from build123d import *

# Parameters (mm, degrees)
CROQUIS1_W              = 158
CROQUIS1_H              = 158
CROQUIS1_W_2            = 146
CROQUIS1_H_2            = 146
SALIENTE_EXTRUIR1_DEPTH = 1.5
CROQUIS2_W              = 150
CROQUIS2_H              = 150
CROQUIS2_W_2            = 146
CROQUIS2_H_2            = 146
SALIENTE_EXTRUIR2_DEPTH = 2


with BuildPart() as part:
    # Croquis1 → Saliente-Extruir1 (new body)
    with BuildSketch(Plane(origin=(0, 0, 0), x_dir=(1, 0, 0), z_dir=(0, 1, 0))):
        with Locations((73, 73)):
            Rectangle(CROQUIS1_W, CROQUIS1_H)
        with Locations((73, 73)):
            Rectangle(CROQUIS1_W_2, CROQUIS1_H_2, mode=Mode.SUBTRACT)
    extrude(amount=SALIENTE_EXTRUIR1_DEPTH)

    # Croquis2 → Saliente-Extruir2 (add)
    with BuildSketch(Plane(origin=(0, 1.5, 0), x_dir=(1, 0, 0), z_dir=(0, 1, 0))):
        with Locations((73, 73)):
            Rectangle(CROQUIS2_W, CROQUIS2_H)
        with Locations((73, 73)):
            Rectangle(CROQUIS2_W_2, CROQUIS2_H_2, mode=Mode.SUBTRACT)
    extrude(amount=SALIENTE_EXTRUIR2_DEPTH)


solid = part.part
Can you work these out from the model? Positions are in its coordinate system, mm. A direction names the side the tool comes from. Coordinates: 2 decimals unless noted, no trailing zeros. Write each loop counter-clockwise with the first axis right and the second up, starting at its lowest first coordinate (ties: lowest second). Pieces come first, ordered by that corner, then holes. Notation, with made-up numbers: (50.5, 48) - (99.5, 48) arc R17 ccw to (99.5, 74) - close; hole circle Ø4 at (81, 26.5). An arc over 180 degrees is marked (long way). Return JSON: item names as keys, results as strings. Group by question number.
Item 1: If we section it at A-A (z = -19.5): Write out the boundary of the cut face in (x, y).
Item 2: We'd pull the mould along Z, two halves only. Please class faces 3 (the face through (72, 2, 0)), 4 (the face through (67, 1.5, 3)): pulls with the +Z half, pulls with the -Z half, needs draft (parallel to the pull), parting line crosses it, or undercut.
Item 3: Which directions (+Z, -Z, +X, -X, +Y, -Y) give clear straight access to the entire face, cutting with the end or side of a thin tool? Please do faces 1 (the face through (146, 2, -72)), 2 (the face through (67, 0, 3)).
Item 4: If we section it at B-B (x = 58): Write out the boundary of the cut face in (y, z), then the cut area to 3 significant figures.
Item 5: Please list where these lines run through material, in increasing order: probe 1 along Z at (x, y) = (26, 1.6); probe 2 along X at (y, z) = (1.35, -38.5); probe 3 along Z at (x, y) = (102, 0.9).
Item 6: I'm going to push flat-ended pins straight in: pin 1 Ø1.5 at (y, z) = (2.5, -53.5) entering from +X; pin 2 Ø1 at (y, z) = (2.5, -48) entering from -X. Where does each tip first touch, or does it pass through?
Item 7: If we section it at C-C (y = 2.35): Write out the boundary of the cut face in (x, z), then the cut area to 3 significant figures.
Return value:
{
 "1": {"outline": "(-6, 0) - (0, 0) - (0, 3.5) - (-2, 3.5) - (-2, 1.5) - (-6, 1.5) - close; (146, 0) - (152, 0) - (152, 1.5) - (148, 1.5) - (148, 3.5) - (146, 3.5) - close"},
 "2": {"face 3": "undercut", "face 4": "needs draft"},
 "3": {"face 1": "+Y, -Y", "face 2": "+Z, -Z, +X, -X, -Y"},
 "4": {"outline": "(0, -152) - (1.5, -152) - (1.5, -148) - (3.5, -148) - (3.5, -146) - (0, -146) - close; (0, 0) - (3.5, 0) - (3.5, 2) - (1.5, 2) - (1.5, 6) - (0, 6) - close", "area": "26.0 mm^2"},
 "5": {"probe 1": "z = -148 to -146, 0 to 2", "probe 2": "x = -6 to 0, 146 to 152", "probe 3": "z = -152 to -146, 0 to 6"},
 "6": {"pin 1": "stops at x = 148", "pin 2": "stops at x = -2"},
 "7": {"outline": "(-2, -148) - (148, -148) - (148, 2) - (-2, 2) - close; hole (0, -146) - (146, -146) - (146, 0) - (0, 0) - close", "area": "1,180 mm^2"}
}
